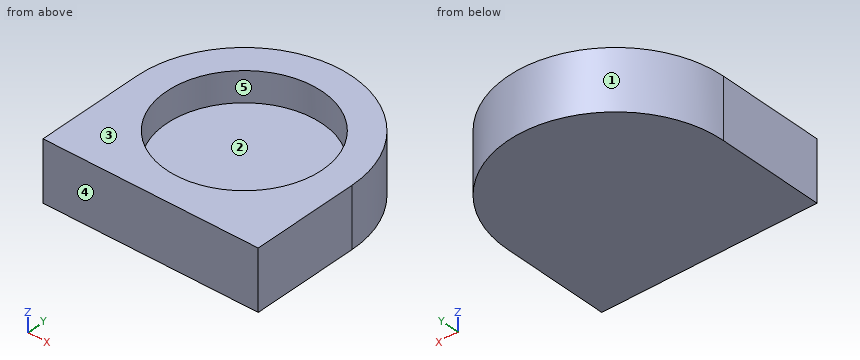
from build123d import *

# Parameters (mm, degrees)
SKETCH_1_R      = 6.5
EXTRUDE_1_DEPTH = 2.5
EXTRUDE_START   = 2.5
EXTRUDE_2_DEPTH = 2.5


with BuildPart() as part:
    # 草图1 → 凸台-拉伸1 (new body)
    with BuildSketch(Plane.XY):
        with BuildLine():
            Line((-9, 0), (-9, -9))
            Line((-9, -9), (9, -9))
            Line((9, -9), (9, 0))
            ThreePointArc((9, 0), (0, 9), (-9, 0))
        make_face()
        Circle(SKETCH_1_R, mode=Mode.SUBTRACT)
    extrude(amount=EXTRUDE_1_DEPTH)

    # 草图2 → 凸台-拉伸2 (add)
    with BuildSketch(Plane(origin=(0, 0, 0), x_dir=(-1, 0, 0), z_dir=(0, 0, -1)).offset(EXTRUDE_START)):
        with BuildLine():
            Line((-9, 0), (-9, -9))
            Line((-9, -9), (9, -9))
            Line((9, -9), (9, 0))
            ThreePointArc((9, 0), (0, 9), (-9, 0))
        make_face()
    extrude(amount=-EXTRUDE_2_DEPTH)


solid = part.part
Here's how the part is built. I have some questions about the finished solid (model axes, mm). Face numbers are marked on the shaded views. A direction names the side the tool comes from. Round coordinates to 2 decimals unless told otherwise and drop trailing zeros. Write each loop counter-clockwise with the first axis right and the second up, starting at its lowest first coordinate (ties: lowest second). Pieces come first, ordered by that corner, then holes. Notation, with made-up numbers: (-15.75, 73) -> (36.25, 73) arc R17 cw to (36.25, 81) -> close; hole circle Ø2 at (-11, 15.5). An arc over 180 degrees is marked (long way). One line per item, written item: value.
1) If I drill on line 1 (X direction, y = -6, z = 0.6); line 2 (Y direction, x = 0, z = 2.1); line 3 (X direction, y = 0.25, z = -1.9), over which ranges is the centre line in solid material (lowest first)? Write a range as [from, to].
Filled sheet:
line 1: x = [-9, -2.5], [2.5, 9]
line 2: y = [-9, -6.5], [6.5, 9]
line 3: x = [-9, 9]
2) Suppose I cut it at D-D on z = -0.95. List the corners of the cut face in (x, y) for me.
Filled sheet:
outline: (-9, -9) -> (9, -9) -> (9, 0) arc R9 ccw to (-9, 0) -> close
3) I'm going to push flat-ended pins straight in: pin 1 Ø1.5 at (x, z) = (6.5, 1) entering from +Y; pin 2 Ø10.5 at (x, y) = (0, 0) entering from +Z. Where does each tip first touch, or does it pass through?
Filled sheet:
pin 1: stops at y = 6.92
pin 2: stops at z = 0
4) For the marked faces 1 and 2, which set-ups out of +Z, -Z, +X, -X, +Y, -Y let a thin tool reach every point of the face, with its end or its side?
Filled sheet:
face 1: +Z, -Z, +Y
face 2: +Z
5) Suppose I cut it at C-C on y = -5.75. List the corners of the cut face in (x, z) for me.
Filled sheet:
outline: (-9, -2.5) -> (9, -2.5) -> (9, 2.5) -> (3.03, 2.5) -> (3.03, 0) -> (-3.03, 0) -> (-3.03, 2.5) -> (-9, 2.5) -> close
6) Suppose I cut it at A-A on x = 0. List the corners of the cut face in (y, z) for me.
Filled sheet:
outline: (-9, -2.5) -> (9, -2.5) -> (9, 2.5) -> (6.5, 2.5) -> (6.5, 0) -> (-6.5, 0) -> (-6.5, 2.5) -> (-9, 2.5) -> close
7) Suppose I cut it at B-B on z = 0.6. List the corners of the cut face in (x, y) for me, plus the area to 3 significant figures.
Filled sheet:
outline: (-9, -9) -> (9, -9) -> (9, 0) arc R9 ccw to (-9, 0) -> close; hole circle Ø13 at (0, 0)
area: 157 mm2
8) We'd pull the mould along Y, two halves only. Please class the marked faces 3, 4 and 5: released by +Y, released by -Y, zero draft, split by the parting line, or undercut.
Filled sheet:
face 3: zero draft
face 4: released by -Y
face 5: undercut
